Autodesk Inventor part; units mm, degrees
ref_plane "to_cp_XY" through (0, 0, 0) normal (1, 0, 0) x (0, 0, -1)
ref_plane "to_cp_YZ" through (0, 0, 0) normal (0, 0, -1) x (0, 1, 0)
ref_plane "to_cp_ZX" through (0, 0, 0) normal (0, 1, 0) x (1, 0, 0)
sketch "Sketch_1" plane through (0, 0, 0) normal (0, 0, 1) x (1, 0, 0)
  line L0 (20, 0) -> (-6, 0)
  line L1 (-6, 0) -> (-6, 4.4)
  line L2 (-6, 4.4) -> (-5.4, 5)
  line L3 (-5.4, 5) -> (0, 5)
  line L4 (0, 5) -> (0, 3)
  line L5 (0, 3) -> (19.3865, 3)
  line L6 (19.3865, 3) -> (20, 2.3865)
  line L7 (20, 2.3865) -> (20, 0)
  line L8 (20, 0) -> (-6, 0)
revolve "Revolution1" add sketch "Sketch_1" angle 360 about axis through (20, 0, 0) along (1, 0, 0)
thread "Thread1"
sketch "Sketch2" plane through (-6, 0, 0) normal (-1, 0, 0) x (0, 0, 1)
  point P0 (0, 0)
hole "Hole1" at (-6, 0, 0) direction (1, 0, 0) diameter 5 depth 3 tip angle 150
sketch "Sketch_3" plane through (-6, 0, 0) normal (1, 0, 0) x (0, 0, -1)
  line L0 (-2.5, -1.4434) -> (0, -2.8868)
  line L1 (0, -2.8868) -> (2.5, -1.4434)
  line L2 (2.5, -1.4434) -> (2.5, 1.4434)
  line L3 (2.5, 1.4434) -> (0, 2.8868)
  line L4 (0, 2.8868) -> (-2.5, 1.4434)
  line L5 (-2.5, 1.4434) -> (-2.5, -1.4434)
extrude "Extrusion1" cut sketch "Sketch_3" along normal blind 3
ref_plane "to_cp_XY" through (0, 0, 0) normal (1, 0, 0) x (0, 0, -1)
ref_plane "to_cp_YZ" through (0, 0, 0) normal (0, 0, -1) x (0, 1, 0)
ref_plane "to_cp_ZX" through (0, 0, 0) normal (0, 1, 0) x (1, 0, 0)
properties part number "BOLT6-20"
Input: part model. Units: mm. Frame: model coordinates. A direction names the side the tool comes from. Give positions to 0.01 mm unless a question says otherwise; leave off trailing zeros. Write each loop counter-clockwise with the first axis right and the second up, starting at its lowest first coordinate (ties: lowest second). Pieces come first, ordered by that corner, then holes. Notation, with made-up numbers: M 87,-3.75 L 114,-3.75 A23 ccw 114,21.25 Z; hole C 10,89.25 d2. An arc over 180 degrees is marked long. Write item = value, one per line. Start each with the question number.
1) Cut plane B-B on x = 10.75. Return the cut outline in (y, z).
2) Draft query along Z for faces 1 (the flat face through (-6, 2, -2)), 2 (the flat face through (-5, 0, 2.5)), 3 (the cylindrical face through (10, -3, 0)). Return one class per face: +Z half, -Z half, draft (parallel to the pull), parting line (faces both ways), or undercut.
3) Cut plane A-A on x = -3.5. Return the cut outline in (y, z).
4) First-contact query: pin 1 Ø4 at (x, z) = (-2.5, -4) entering from +Y; pin 2 Ø6 at (x, z) = (14.5, 2) entering from -Y; pin 3 Ø2 at (x, y) = (7, 0) entering from +Z. Flat tips, straight axial feed; report the tip coordinate or a pass-through.
5) Reachability of faces 4 (the flat face through (0, 3.3, 0.1)), 5 (the flat face through (20, 0, 0)), 6 (the flat face through (-4.521, 2.175, 1.233)) from +Z, -Z, +X, -X, +Y, -Y: full face, straight path, thin tool, end or side. Return the list, or none.
6) Material intervals for line 1 along X through (y, z) = (-3.75, -2.25); line 2 along Z through (x, y) = (7.5, 0); line 3 along Y through (x, z) = (-3.75, 0.75), sorted ascending. Write a range as [from, to].
Solved:
q1.outline = C 0,0 d6
q2.face_1 = draft
q2.face_2 = undercut
q2.face_3 = parting line
q3.outline = C 0,0 d10; hole M -2.89,0 L -1.44,-2.5 L 1.44,-2.5 L 2.89,0 L 1.44,2.5 L -1.44,2.5 Z
q4.pin_1 = 4.58
q4.pin_2 = -3
q4.pin_3 = 3
q5.face_4 = +X
q5.face_5 = +Z, -Z, +X, +Y, -Y
q5.face_6 = -X
q6.line_1 = [-6, 0]
q6.line_2 = [-3, 3]
q6.line_3 = [-4.94, -2.45], [2.45, 4.94]
